```python
from build123d import *

# Parameters (mm, degrees)
F0_R     = 10
F1_DEPTH = 20
F2_R     = 11.9866247271
F3_DEPTH = 2
F4_R     = 0.99999
F6_DEPTH = 1


# Not quite as in the source:
# - a fillet or chamfer is up to 0.001 mm smaller than in the source, because OpenCascade refuses the exact size


with BuildPart() as f1:
    # F0 (on Front) → F1 (new body)
    with BuildSketch(Plane.XZ):
        with BuildLine():
            Line((6.9282032303, 15), (-6.9282032303, 15))
            ThreePointArc((-6.9282032303, 15), (-8.4282032303, 14.5980762114), (-9.5262794416, 13.5))
            Line((-9.5262794416, 13.5), (-16.4544826719, 1.5))
            ThreePointArc((-16.4544826719, 1.5), (-16.8564064606, 0), (-16.4544826719, -1.5))
            Line((-16.4544826719, -1.5), (-9.5262794416, -13.5))
            ThreePointArc((-9.5262794416, -13.5), (-8.4282032303, -14.5980762114), (-6.9282032303, -15))
            Line((-6.9282032303, -15), (6.9282032303, -15))
            ThreePointArc((6.9282032303, -15), (8.4282032303, -14.5980762114), (9.5262794416, -13.5))
            Line((9.5262794416, -13.5), (16.4544826719, -1.5))
            ThreePointArc((16.4544826719, -1.5), (16.8564064606, 0), (16.4544826719, 1.5))
            Line((16.4544826719, 1.5), (9.5262794416, 13.5))
            ThreePointArc((9.5262794416, 13.5), (8.4282032303, 14.5980762114), (6.9282032303, 15))
        make_face()
        Circle(F0_R, mode=Mode.SUBTRACT)
    extrude(amount=F1_DEPTH)

    # F2 (on face) → F3 (join)
    with BuildSketch(Plane.XZ.offset(20)):
        Circle(F2_R)
    extrude(amount=F3_DEPTH)

    # F4 (radius 1 in the source; OpenCascade refuses exactly that, so slightly less here)
    f4_edges = [f1.edges().sort_by_distance(p)[0] for p in [
        (-11.986625, -22, 0),
        (-11.986625, -20, 0),
    ]]
    fillet(f4_edges, radius=F4_R)

    # F5 (on face) → F6 (cut)
    with BuildSketch(Plane.XZ.offset(22)):
        Polygon((3.027519893, 5.2438182756), (-3.027519893, 5.2438182756), (-6.055039786, 0), (-3.027519893, -5.2438182756), (3.027519893, -5.2438182756), (6.055039786, 0), align=None)
    extrude(amount=-F6_DEPTH, mode=Mode.SUBTRACT)


solid = f1.part
```
CAD build for the part. Positions are in the model's coordinates, mm. A direction names the side the tool comes from. Round coordinates to 2 decimals unless told otherwise and drop trailing zeros. Write each loop counter-clockwise with the first axis right and the second up, starting at its lowest first coordinate (ties: lowest second). Pieces come first, ordered by that corner, then holes. Notation, with made-up numbers: (-20, -2.75) -> (19, -2.75) arc R35 cw to (19, 34.25) -> close; hole circle Ø2 at (-31.5, -29.5). An arc over 180 degrees is marked (long way). Answer in a Markdown table with one row per item. Add a question column.
Item 1: Mould opens along Z. For faces 1 (the face through (0, -10, -15)), 2 (the face through (0, -21.5, 5.244)), 3 (the face through (13.039, -9.86, 7.416)) say: pulls with the +Z half, pulls with the -Z half, needs draft (parallel to the pull), parting line crosses it, or undercut.
Item 2: Drill centre lines: line 1 (Z direction, x = 0, y = -5); line 2 (X direction, y = -4.75, z = -0.25); line 3 (Y direction, x = 9.5, z = -10). Where is each one in solid material? Low to high. Write a range as from..to.
Item 3: Saw through at C-C, the plane x = 15. Write the cut outline in (y, z), then the cut area to 3 significant figures.
Item 4: Saw through at A-A, the plane y = -14. Write the cut outline in (x, z), then the cut area to 3 significant figures.
Item 5: Drop flat-ended pins along their axis: pin 1 Ø5 at (y, z) = (-16, 5) entering from -X; pin 2 Ø10 at (x, y) = (-13.5, -16.5) entering from -Z; pin 3 Ø0.8 at (x, y) = (0.5, -21.5) entering from +Z. Give the stop position or say it passes through.
Item 6: Which spindle directions (+Z, -Z, +X, -X, +Y, -Y) get a long thin tool onto all of the face, cutting with end or side? Do faces 4 (the face through (0, -20, 0)), 5 (the face through (-13, -20, 3)), 6 (the face through (-13.039, -9.86, -7.416)). Say none if no direction does.
Findings below:
| question | item | result |
|---|---|---|
| 1 | face 1 | pulls with the -Z half |
| 1 | face 2 | undercut |
| 1 | face 3 | pulls with the +Z half |
| 2 | line 1 | z = -15..-10, 10..15 |
| 2 | line 2 | x = -16.85..-10, 10..16.85 |
| 2 | line 3 | y = -20..0 |
| 3 | outline | (-20, -4.02) -> (0, -4.02) -> (0, 4.02) -> (-20, 4.02) -> close |
| 3 | area | 161 mm^2 |
| 4 | outline | (-16.45, -1.5) -> (-9.53, -13.5) arc R3 ccw to (-6.93, -15) -> (6.93, -15) arc R3 ccw to (9.53, -13.5) -> (16.45, -1.5) arc R3 ccw to (16.45, 1.5) -> (9.53, 13.5) arc R3 ccw to (6.93, 15) -> (-6.93, 15) arc R3 ccw to (-9.53, 13.5) -> (-16.45, 1.5) arc R3 ccw to start; hole circle Ø20 at (0, 0) |
| 4 | area | 462 mm^2 |
| 5 | pin 1 | stops at x = -15.88 |
| 5 | pin 2 | stops at z = -14.56 |
| 5 | pin 3 | stops at z = 11.97 |
| 6 | face 4 | +Y |
| 6 | face 5 | -Y |
| 6 | face 6 | -Z, -X, +Y, -Y |
